Geometry: final body of the model. Coordinates: model frame, mm. Coordinates: 2 decimals unless noted, no trailing zeros. Order: outer loops, then holes, each group sorted by start corner. A loop starts at its lowest first (then second) coordinate and runs counter-clockwise, first axis right, second up. Notation, with made-up numbers: M 69.5,46 L 126.5,46 A21 ccw 126.5,56 Z; hole C 20.5,-20 d5. An arc over 180 degrees is marked long. Write item = value, one per line.
from build123d import *

# Parameters (mm, degrees)
F0_W     = 200
F0_H     = 145
F0_R     = 2
F0_W_2   = 10
F0_H_2   = 3
F0_R_2   = 1.5
F0_W_3   = 3
F0_H_3   = 10
F0_H_4   = 135
F1_DEPTH = 3


with BuildPart() as f1:
    # F0 (on Top) → F1 (new body)
    with BuildSketch(Plane.XY):
        with Locations((42.636041, 49.168777)):
            Rectangle(F0_W, F0_H)
        with Locations((-43.113959, 14.168777)):
            Circle(F0_R, mode=Mode.SUBTRACT)
        with Locations((-16.363959, -18.331223)):
            Rectangle(F0_W_2, F0_H_2, mode=Mode.SUBTRACT)
        with Locations((-4.863959, -18.331223)):
            Circle(F0_R_2, mode=Mode.SUBTRACT)
        with Locations((6.636041, -18.331223)):
            Rectangle(F0_W_2, F0_H_2, mode=Mode.SUBTRACT)
        with BuildLine():
            ThreePointArc((-28.34783, 13.408052), (-28.054936, 14.115159), (-27.34783, 14.408052))
            Line((-27.34783, 14.408052), (10.75808, 14.408052))
            ThreePointArc((10.75808, 14.408052), (11.465186, 14.115159), (11.75808, 13.408052))
            Line((11.75808, 13.408052), (11.75808, -3.846393))
            ThreePointArc((11.75808, -3.846393), (11.465186, -4.553499), (10.75808, -4.846393))
            Line((10.75808, -4.846393), (-27.34783, -4.846393))
            ThreePointArc((-27.34783, -4.846393), (-28.054936, -4.553499), (-28.34783, -3.846393))
            Line((-28.34783, -3.846393), (-28.34783, 13.408052))
        make_face(mode=Mode.SUBTRACT)
        with Locations((-52.365544, 37.668777)):
            Rectangle(F0_W_3, F0_H_3, mode=Mode.SUBTRACT)
        with Locations((-52.363959, 49.168777)):
            Circle(F0_R_2, mode=Mode.SUBTRACT)
        with Locations((-7.363959, 32.668777)):
            Circle(F0_R, mode=Mode.SUBTRACT)
        with Locations((78.636041, -18.331223)):
            Rectangle(F0_W_2, F0_H_2, mode=Mode.SUBTRACT)
        with Locations((90.136041, -18.331223)):
            Circle(F0_R_2, mode=Mode.SUBTRACT)
        Polygon((78.136041, 32.168777), (81.136041, 32.168777), (81.136041, 3.668777), (89.636041, 3.668777), (89.636041, 0.668777), (81.136041, 0.668777), (81.136041, -7.831223), (78.136041, -7.831223), (78.136041, 0.668777), (64.636041, 0.668777), (64.636041, 3.668777), (78.136041, 3.668777), align=None, mode=Mode.SUBTRACT)
        with Locations((32.636041, 32.668777)):
            Circle(F0_R, mode=Mode.SUBTRACT)
        with Locations((68.636041, 46.668777)):
            Rectangle(F0_W_2, F0_H_2, mode=Mode.SUBTRACT)
        with Locations((80.136041, 46.668777)):
            Circle(F0_R_2, mode=Mode.SUBTRACT)
        with Locations((-52.365544, 60.668777)):
            Rectangle(F0_W_3, F0_H_3, mode=Mode.SUBTRACT)
        with Locations((-43.113959, 84.168777)):
            Circle(F0_R, mode=Mode.SUBTRACT)
        with Locations((-7.363959, 65.668777)):
            Circle(F0_R, mode=Mode.SUBTRACT)
        with BuildLine():
            Line((-27.34783, 103.183946), (10.75808, 103.183946))
            ThreePointArc((10.75808, 103.183946), (11.465186, 102.891053), (11.75808, 102.183946))
            Line((11.75808, 102.183946), (11.75808, 84.929501))
            ThreePointArc((11.75808, 84.929501), (11.465186, 84.222394), (10.75808, 83.929501))
            Line((10.75808, 83.929501), (-27.34783, 83.929501))
            ThreePointArc((-27.34783, 83.929501), (-28.054936, 84.222394), (-28.34783, 84.929501))
            Line((-28.34783, 84.929501), (-28.34783, 102.183946))
            ThreePointArc((-28.34783, 102.183946), (-28.054936, 102.891053), (-27.34783, 103.183946))
        make_face(mode=Mode.SUBTRACT)
        with Locations((-16.363959, 116.668777)):
            Rectangle(F0_W_2, F0_H_2, mode=Mode.SUBTRACT)
        with Locations((-4.863959, 116.668777)):
            Circle(F0_R_2, mode=Mode.SUBTRACT)
        with Locations((6.636041, 116.668777)):
            Rectangle(F0_W_2, F0_H_2, mode=Mode.SUBTRACT)
        with Locations((22.634456, 70.168777)):
            Rectangle(F0_W_3, F0_H_3, mode=Mode.SUBTRACT)
        with Locations((32.636041, 65.668777)):
            Circle(F0_R, mode=Mode.SUBTRACT)
        with Locations((22.636041, 81.668777)):
            Circle(F0_R_2, mode=Mode.SUBTRACT)
        Polygon((81.136041, 94.668777), (81.136041, 66.168777), (78.136041, 66.168777), (78.136041, 94.668777), (64.636041, 94.668777), (64.636041, 97.668777), (78.136041, 97.668777), (78.136041, 106.168777), (81.136041, 106.168777), (81.136041, 97.668777), (89.636041, 97.668777), (89.636041, 94.668777), align=None, mode=Mode.SUBTRACT)
        with Locations((22.634456, 93.168777)):
            Rectangle(F0_W_3, F0_H_3, mode=Mode.SUBTRACT)
        with Locations((78.636041, 116.668777)):
            Rectangle(F0_W_2, F0_H_2, mode=Mode.SUBTRACT)
        with Locations((90.136041, 116.668777)):
            Circle(F0_R_2, mode=Mode.SUBTRACT)
        with Locations((101.636041, -18.331223)):
            Rectangle(F0_W_2, F0_H_2, mode=Mode.SUBTRACT)
        with Locations((99.636041, 2.168777)):
            Circle(F0_R_2, mode=Mode.SUBTRACT)
        Polygon((118.136041, 3.668777), (118.136041, 32.168777), (121.136041, 32.168777), (121.136041, 3.668777), (126.136041, 3.668777), (126.136041, 0.668777), (121.136041, 0.668777), (121.136041, -7.831223), (118.136041, -7.831223), (118.136041, 0.668777), (109.636041, 0.668777), (109.636041, 3.668777), align=None, mode=Mode.SUBTRACT)
        with Locations((91.636041, 46.668777)):
            Rectangle(F0_W_2, F0_H_2, mode=Mode.SUBTRACT)
        with Locations((137.636041, 49.168777)):
            Rectangle(F0_W_3, F0_H_4, mode=Mode.SUBTRACT)
        Polygon((118.136041, 97.668777), (118.136041, 106.168777), (121.136041, 106.168777), (121.136041, 97.668777), (126.136041, 97.668777), (126.136041, 94.668777), (121.136041, 94.668777), (121.136041, 66.168777), (118.136041, 66.168777), (118.136041, 94.668777), (109.636041, 94.668777), (109.636041, 97.668777), align=None, mode=Mode.SUBTRACT)
        with Locations((99.636041, 96.168777)):
            Circle(F0_R_2, mode=Mode.SUBTRACT)
        with Locations((101.636041, 116.668777)):
            Rectangle(F0_W_2, F0_H_2, mode=Mode.SUBTRACT)
    extrude(amount=F1_DEPTH)


solid = f1.part
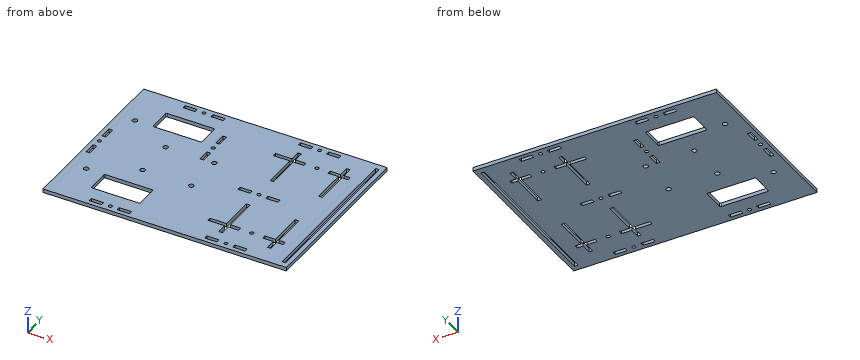
1) Line query: L1, parallel to X at y = 9, z = 0.3; L2, parallel to Y at x = -17, z = 1.4; L3, parallel to X at y = 42.5, z = 2.3. Output: solid intervals per line, ascending.
Numbers:
L1 = -57.36 to -28.35, 11.76 to 78.14, 81.14 to 118.14, 121.14 to 136.14, 139.14 to 142.64
L2 = -23.33 to -19.83, -16.83 to -4.85, 14.41 to 83.93, 103.18 to 115.17, 118.17 to 121.67
L3 = -57.36 to -53.87, -50.87 to 136.14, 139.14 to 142.64
2) Section D-D, the plane z = 2. Give the number of separate pieces and of enclosed holes in the cut face, and give its area (3 significant figures).
Numbers:
separate_pieces = 1
enclosed_holes = 36
area = 25,800 mm²
3) Section C-C, the plane y = 70. Return loops of the section in (x, z).
Numbers:
outline = M -57.36,0 L 21.13,0 L 21.13,3 L -57.36,3 Z; M 24.13,0 L 78.14,0 L 78.14,3 L 24.13,3 Z; M 81.14,0 L 118.14,0 L 118.14,3 L 81.14,3 Z; M 121.14,0 L 136.14,0 L 136.14,3 L 121.14,3 Z; M 139.14,0 L 142.64,0 L 142.64,3 L 139.14,3 Z
4) Section B-B, the plane x = 7. Return loops of the section in (y, z), and give its area (3 significant figures).
Numbers:
outline = M -23.33,0 L -19.83,0 L -19.83,3 L -23.33,3 Z; M -16.83,0 L -4.85,0 L -4.85,3 L -16.83,3 Z; M 14.41,0 L 83.93,0 L 83.93,3 L 14.41,3 Z; M 103.18,0 L 115.17,0 L 115.17,3 L 103.18,3 Z; M 118.17,0 L 121.67,0 L 121.67,3 L 118.17,3 Z
area = 301 mm²
5) Section A-A, the plane y = 26.5. Return loops of the section in (x, z).
Numbers:
outline = M -57.36,0 L 78.14,0 L 78.14,3 L -57.36,3 Z; M 81.14,0 L 118.14,0 L 118.14,3 L 81.14,3 Z; M 121.14,0 L 136.14,0 L 136.14,3 L 121.14,3 Z; M 139.14,0 L 142.64,0 L 142.64,3 L 139.14,3 Z
